Work out the finished part from the listing and answer in its coordinate system (mm). Give positions to 0.01 mm unless a question says otherwise; leave off trailing zeros. Loops run counter-clockwise (first coordinate to the right, second up) from the corner with the lowest first, then second, coordinate; pieces in that order, holes last. Notation, with made-up numbers: (24.5, 21) - (47.5, 21) arc R18 cw to (47.5, 51) - close; hole circle Ø11 at (56, 72). An arc over 180 degrees is marked (long way). Use CSV: the item, a comma, the result in double quotes.
from build123d import *

# Parameters (mm, degrees)
SZKIC1_W                    = 111
SZKIC1_H                    = 90
DODANIE_WYCI_GNI_CIE1_DEPTH = 3
SZKIC2_R                    = 2.1
WYTNIJ_WYCI_GNI_CIE2_DEPTH  = 143.933550995
SZKIC3_R                    = 3.1
SZKIC3_R_2                  = 2.1
WYTNIJ_WYCI_GNI_CIE3_DEPTH  = 143.933550995


with BuildPart() as part:
    # Szkic1 → Dodanie-wyciągnięcie1 (new body)
    with BuildSketch(Plane.XY):
        with Locations((55.5, 45)):
            Rectangle(SZKIC1_W, SZKIC1_H)
    extrude(amount=DODANIE_WYCI_GNI_CIE1_DEPTH)

    # Szkic2 → Wytnij-wyciągnięcie2 (cut, through all)
    with BuildSketch(Plane.XY.offset(3)):
        with Locations((18.05, 24)):
            Circle(SZKIC2_R)
        with Locations((18.05, 10)):
            Circle(SZKIC2_R)
        with Locations((92.75, 24)):
            Circle(SZKIC2_R)
        with Locations((92.75, 10)):
            Circle(SZKIC2_R)
    extrude(amount=-WYTNIJ_WYCI_GNI_CIE2_DEPTH, mode=Mode.SUBTRACT)

    # Szkic3 → Wytnij-wyciągnięcie3 (cut, through all)
    with BuildSketch(Plane.XY.offset(3)):
        with Locations((93, 82)):
            Circle(SZKIC3_R)
        with Locations((93, 42)):
            Circle(SZKIC3_R_2)
        with Locations(Location((18, 42, 0), (0, 0, 180))):
            Circle(SZKIC3_R_2)
        with Locations(Location((18, 82, 0), (0, 0, 180))):
            Circle(SZKIC3_R)
    extrude(amount=-WYTNIJ_WYCI_GNI_CIE3_DEPTH, mode=Mode.SUBTRACT)


solid = part.part
Item 1: The mould has two halves that part along Y. Classify faces 1 (the flat face through (55, 0, 1)), 2 (the flat face through (55, 46, 3)), 3 (the flat face through (55, 90, 1)), 4 (the cylindrical face through (17.777, 26.082, 1.521)): pulls with the +Y half, pulls with the -Y half, needs draft (parallel to the pull), parting line crosses it, or undercut.
Determined:
face 1,"pulls with the -Y half"
face 2,"needs draft"
face 3,"pulls with the +Y half"
face 4,"undercut"
Item 2: A cutting plane is placed at C-C on y = 24. Determine the outline of the cut face in (x, z), and give its area (3 significant figures).
Determined:
outline,"(0, 0) - (15.95, 0) - (15.95, 3) - (0, 3) - close; (20.15, 0) - (90.65, 0) - (90.65, 3) - (20.15, 3) - close; (94.85, 0) - (111, 0) - (111, 3) - (94.85, 3) - close"
area,"308 mm²"
Item 3: Find the intervals of material crossed by line 1 (Y direction, x = 92.75, z = 1); line 2 (X direction, y = 11.5, z = 1.4), in increasing order.
Determined:
line 1,"y = 0 to 7.9, 12.1 to 21.9, 26.1 to 39.91, 44.09 to 78.91, 85.09 to 90"
line 2,"x = 0 to 16.58, 19.52 to 91.28, 94.22 to 111"
Item 4: A cutting plane is placed at B-B on x = 93. Determine the outline of the cut face in (y, z).
Determined:
outline,"(0, 0) - (7.91, 0) - (7.91, 3) - (0, 3) - close; (12.09, 0) - (21.91, 0) - (21.91, 3) - (12.09, 3) - close; (26.09, 0) - (39.9, 0) - (39.9, 3) - (26.09, 3) - close; (44.1, 0) - (78.9, 0) - (78.9, 3) - (44.1, 3) - close; (85.1, 0) - (90, 0) - (90, 3) - (85.1, 3) - close"
Item 5: Given P1, Ø5.5, axis at x = 93, y = 42, coming from the -Z side, flat-ended and moving along its own axis, determine where the tip first touches the part or whether it passes through.
Determined:
P1,"stops at z = 0"
Item 6: A cutting plane is placed at A-A on y = 82. Determine the outline of the cut face in (x, z), and give its area (3 significant figures).
Determined:
outline,"(0, 0) - (14.9, 0) - (14.9, 3) - (0, 3) - close; (21.1, 0) - (89.9, 0) - (89.9, 3) - (21.1, 3) - close; (96.1, 0) - (111, 0) - (111, 3) - (96.1, 3) - close"
area,"296 mm²"
